Autodesk Inventor part; units mm, degrees
ref_plane "YZ Plane" through (0, 0, 0) normal (1, 0, 0) x (0, 1, 0)
ref_plane "XZ Plane" through (0, 0, 0) normal (0, 1, 0) x (-1, 0, 0)
ref_plane "XY Plane" through (0, 0, 0) normal (0, 0, 1) x (1, 0, 0)
sketch "Sketch1" plane through (0, 0, 0) normal (0, 1, 0) x (-1, 0, 0)
  circle A0 centre (0, 0) radius 12.5
  dimension "d0" = 25
extrude "Extrusion1" add sketch "Sketch1" along normal blind 30
hole "ReliefTop" at (0, 30, 0) direction (0, -1, 0) diameter 13.97 depth 0.254 countersink diameter 14.478 countersink angle 90
hole "ReliefBottom" at (0, 0, 0) direction (0, 1, 0) diameter 13.97 depth 0.254 countersink diameter 14.478 countersink angle 90
hole "MountBottomM6" at (0, 0.254, 0) direction (0, 1, 0) diameter 4.917 depth 7.366 tip angle 118 countersink diameter 5.508 countersink angle 90
hole "MountTopM4" at (0, 29.746, 0) direction (0, -1, 0) diameter 3.242 depth 14.478 tip angle 118 countersink diameter 3.808 countersink angle 90
sketch "Sketch2" plane through (0, 0, 0) normal (0, 0, 1) x (1, 0, 0)
  circle A0 centre (0, 20) radius 3
  line L0 (-12.5, 0) -> (12.5, 0)
  line L1 (0, -4.6) -> (0, 27.6)
  point P0 (0, 0)
  dimension "d49" = 6
  dimension "d50" = 20
extrude "Extrusion2" cut sketch "Sketch2" along normal through all both and the other way through all
chamfer "Chamfer1" distance 0.313 angle 45 2 edges at (-3, 19.9998, 12.1347) (-3, 19.9998, -12.1347)
extrude "Extrusion3" add sketch "Sketch2" along normal mid plane 14.84
equation "\"d1\" = height"
equation "\"d5\" = reliefMinor"
equation "\"d7\" = reliefMajor"
equation "\"d10\" = reliefDepth"
equation "\"d14\" = reliefMinor"
equation "\"d16\" = reliefMajor"
equation "\"d19\" = reliefDepth"
equation "\"d25\" = chamferM6"
equation "\"d28\" = depthM6"
equation "\"d40\" = chamferM4"
equation "\"d43\" = depthM4"
equation "\"reliefDepth\" = 0.254"
equation "\"reliefMinor\" = 13.97"
equation "\"reliefMajor\" = 14.478"
equation "\"chamferM6\" = 5.508"
equation "\"chamferM4\" = 3.808"
equation "\"depthM6\" = 7.366"
equation "\"depthM4\" = 14.478"
equation "\"height\" = 30"
properties part number "PLS-P642H0300A00_M" material "Stainless Steel"
The model under review builds one solid part; all positions refer to its coordinate system, in mm. A direction names the side the tool comes from. Round coordinates to 2 decimals unless told otherwise and drop trailing zeros. Write each loop counter-clockwise with the first axis right and the second up, starting at its lowest first coordinate (ties: lowest second). Pieces come first, ordered by that corner, then holes. Notation, with made-up numbers: (-38, 79) - (-32, 79) arc R11 cw to (-32, 92) - close; hole circle Ø7 at (40, 80.5). An arc over 180 degrees is marked (long way). Use one line per item in the form item = value.
Q1. Consider section B-B (z = -8). State the section outline as (x, y) points.
Answer key:
outline = (-9.6, 0) - (9.6, 0) - (9.6, 30) - (-9.6, 30) - close; hole circle Ø6 at (0, 20)
Q2. Consider section D-D (x = -9). State the section outline as (y, z) points.
Answer key:
outline = (0, -8.67) - (30, -8.67) - (30, 8.67) - (0, 8.67) - close
Q3. Draft analysis for pull direction Z (two halves, no side actions). For faces 1 (the cylindrical face through (-0.07, 25.95, -1.62)), 2 (the flat face through (0, 20, 7.42)), 3 (the flat face through (0, 20, -7.42)), 4 (the cylindrical face through (-11.923, 14.79, -3.755)), state which applies: +Z half, -Z half, draft (parallel to the pull), parting line (faces both ways), or undercut.
Answer key:
face_1 = undercut
face_2 = +Z half
face_3 = -Z half
face_4 = parting line
Q4. Consider section C-C (y = 28.5). State the section outline as (x, z) points, and give its area (3 significant figures).
Answer key:
outline = circle Ø25 at (0, 0); hole circle Ø3.24 at (0, 0)
area = 483 mm2
Q5. Insertion check: pin 1 Ø12 at (y, z) = (13.5, -1) entering from -X; pin 2 Ø1 at (x, z) = (-2, 2) entering from -Y; pin 3 Ø6 at (y, z) = (26, -9.5) entering from +X; pin 4 Ø7 at (x, z) = (-1, 1.5) entering from +Y. Each pin has a flat end and moves straight along its axis. Give the tip position at first contact, or say it passes through.
Answer key:
pin_1 = -12.5
pin_2 = 0.25
pin_3 = 10.68
pin_4 = 29.75
Q6. Consider section A-A (y = 6). State the section outline as (x, z) points.
Answer key:
outline = circle Ø25 at (0, 0); hole circle Ø4.92 at (0, 0)
Q7. For line 1 (Y direction, x = 0, z = -9.5); line 2 (X direction, y = 2, z = -0.5); line 3 (X direction, y = 19, z = -2.75), list the stretches that pass through material, from the lowest coordinate up. Write a range as [from, to].
Answer key:
line_1 = [0, 17], [23, 30]
line_2 = [-12.49, -2.41], [2.41, 12.49]
line_3 = [-12.19, 12.19]
Q8. Tool access review of faces 5 (the flat face through (1.5, 29.746, 1.5)), 6 (the flat face through (0, 0.254, -3)), 7 (the cylindrical face through (0, 23, 10)), 8 (the conical face through (-0.27, 14.46, -0.06)), 9 (the cylindrical face through (-3, 20, -10)): name each direction out of +Z, -Z, +X, -X, +Y, -Y from which nothing blocks a thin tool from reaching the whole face with its end or side.
Answer key:
face_5 = +Y
face_6 = -Y
face_7 = +Z
face_8 = none
face_9 = -Z
